Geometry: final body of the model. Coordinates: model frame, mm. Face numbers are marked on the shaded views. A direction names the side the tool comes from. Give positions to 0.01 mm unless a question says otherwise; leave off trailing zeros. Order: outer loops, then holes, each group sorted by start corner. A loop starts at its lowest first (then second) coordinate and runs counter-clockwise, first axis right, second up. Notation, with made-up numbers: (89.5, 13.5) -> (103.5, 13.5) arc R27 ccw to (103.5, 40.5) -> close; hole circle Ø10 at (-36.5, 23). An arc over 180 degrees is marked (long way). One line per question, with ' | ' between items.
from build123d import *

# Parameters (mm, degrees)
ESBO_O1_R                  = 72.5
ESBO_O1_R_2                = 52.5
RESSALTO_EXTRUS_O1_DEPTH   = 50
CORTE_EXTRUS_O1_DEPTH      = 115.072345465
CORTE_EXTRUS_O1_DEPTH_BACK = 115.072345465
ESBO_O2_W                  = 40
ESBO_O2_H                  = 97.356983932
RESSALTO_EXTRUS_O2_START   = -30
ESBO_O3_R                  = 52.5
ESBO_O3_R_2                = 47.8
RESSALTO_EXTRUS_O2_DEPTH   = 30
CORTE_EXTRUS_O2_DEPTH      = 115.072345465
CORTE_EXTRUS_O2_DEPTH_BACK = 115.072345465
ESBO_O5_W                  = 23.143765799
ESBO_O5_H                  = 26
CORTE_EXTRUS_O3_DEPTH      = 115.072345465


with BuildPart() as part:
    # Esboço1 → Ressalto-extrusão1 (new body)
    with BuildSketch(Plane(origin=(0, 0, 0), x_dir=(1, 0, 0), z_dir=(0, 1, 0))):
        with Locations(Location((0, 0, 0), (0, 0, 270))):
            Circle(ESBO_O1_R)
        with Locations(Location((0, 0, 0), (0, 0, 270))):
            Circle(ESBO_O1_R_2, mode=Mode.SUBTRACT)
    extrude(amount=RESSALTO_EXTRUS_O1_DEPTH)

    # Esboço2 → Corte-extrusão1 (cut, two sides: drawn at the far end of the back side and taken through both)
    with BuildSketch(Plane(origin=(0, 50, 0), x_dir=(1, 0, 0), z_dir=(0, 1, 0)).offset(-CORTE_EXTRUS_O1_DEPTH_BACK)):
        with Locations((0, 48.678491966)):
            Rectangle(ESBO_O2_W, ESBO_O2_H)
    extrude(amount=CORTE_EXTRUS_O1_DEPTH + CORTE_EXTRUS_O1_DEPTH_BACK, mode=Mode.SUBTRACT)

    # Esboço3 → Ressalto-extrusão2 (add)
    with BuildSketch(Plane(origin=(0, 50, 0), x_dir=(1, 0, 0), z_dir=(0, 1, 0)).offset(RESSALTO_EXTRUS_O2_START)):
        Circle(ESBO_O3_R)
        with Locations(Location((0, 0, 0), (0, 0, 270))):
            Circle(ESBO_O3_R_2, mode=Mode.SUBTRACT)
    extrude(amount=RESSALTO_EXTRUS_O2_DEPTH)

    # Esboço4 → Corte-extrusão2 (cut, two sides: drawn at the far end of the back side and taken through both)
    with BuildSketch(Plane(origin=(0, 50, 0), x_dir=(1, 0, 0), z_dir=(0, 1, 0)).offset(-CORTE_EXTRUS_O2_DEPTH_BACK)):
        Polygon((-20, 69.686799324), (-20, 29.755386526), (20, 29.755386526), (20, 73.66525197), (-20, 73.66525197), align=None)
    extrude(amount=CORTE_EXTRUS_O2_DEPTH + CORTE_EXTRUS_O2_DEPTH_BACK, mode=Mode.SUBTRACT)

    # Esboço5 → Corte-extrusão3 (cut, through all)
    with BuildSketch(Plane(origin=(0, 0, 0), x_dir=(0, 0, -1), z_dir=(1, 0, 0))):
        with Locations((-61.895664133, 33.904990218)):
            Rectangle(ESBO_O5_W, ESBO_O5_H)
    extrude(amount=-CORTE_EXTRUS_O3_DEPTH, mode=Mode.SUBTRACT)


solid = part.part
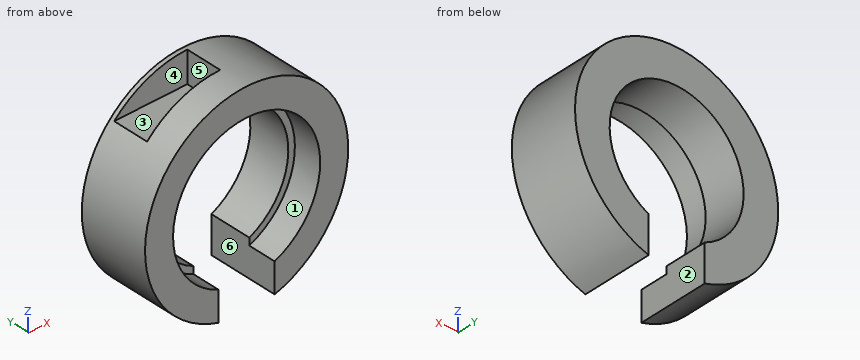
1) Section B-B on y = 44.5. Return loops of the section in (x, z), plus the area to 3 significant figures.
Check result:
outline: (-52.19, 50.32) arc R72.5 ccw to (-20, -69.69) -> (-20, -43.41) arc R47.8 cw (long way) to (20, -43.41) -> (20, -69.69) arc R72.5 ccw to (0, 72.5) -> (0, 50.32) -> close | area: 7,530 mm^2
2) Pull-direction query (X, two-part tool) for the marked faces 4, 5 and 6; classes: +X half, -X half, draft (parallel to the pull), parting line (faces both ways), or undercut.
Check result:
face 4: draft | face 5: -X half | face 6: undercut
3) Contact query for flat-ended pins moving along their axis: pin 1 Ø8 at (y, z) = (18.5, -50.5) entering from +X; pin 2 Ø10 at (x, y) = (-4, 28) entering from +Z; pin 3 Ø6 at (y, z) = (36, -17) entering from +X; pin 4 Ø6 at (x, y) = (5.5, 6) entering from -Z. Output: stop coordinate, or through.
Check result:
pin 1: stops at x = 55.62 | pin 2: stops at z = 72.5 | pin 3: stops at x = 71.14 | pin 4: stops at z = 51.81
4) Section D-D on z = 39.5. Return loops of the section in (x, y), plus the area to 3 significant figures.
Check result:
outline: (-60.79, 0) -> (-34.58, 0) -> (-34.58, 20) -> (-26.92, 20) -> (-26.92, 50) -> (-60.79, 50) -> close; (26.92, 20) -> (34.58, 20) -> (34.58, 0) -> (60.79, 0) -> (60.79, 50) -> (26.92, 50) -> close | area: 3,080 mm^2
5) Section A-A on z = 0. Return loops of the section in (x, y).
Check result:
outline: (-72.5, 0) -> (-52.5, 0) -> (-52.5, 20) -> (-47.8, 20) -> (-47.8, 50) -> (-72.5, 50) -> close; (47.8, 20) -> (52.5, 20) -> (52.5, 0) -> (72.5, 0) -> (72.5, 50) -> (47.8, 50) -> close
6) Material intervals for probe 1 along X at (y, z) = (39.5, 0); probe 2 along X at (y, z) = (12, 0); probe 3 along Z at (x, y) = (0, 16.25), sorted ascending. Write a range as from..to.
Check result:
probe 1: x = -72.5..-47.8, 47.8..72.5 | probe 2: x = -72.5..-52.5, 52.5..72.5 | probe 3: z = 52.5..72.5
7) Section C-C on x = -28. Return loops of the section in (y, z) (3 decimals).
Check result:
outline: (0, -66.875) -> (50, -66.875) -> (50, -38.741) -> (20, -38.741) -> (20, -44.41) -> (0, -44.41) -> close; (0, 44.41) -> (20, 44.41) -> (20, 38.741) -> (50, 38.741) -> (50, 66.875) -> (46.905, 66.875) -> (46.905, 50.324) -> (20.905, 50.324) -> (20.905, 66.875) -> (0, 66.875) -> close
8) Set-up query: the marked faces 1, 2 and 3. Return all of +Z, -Z, +X, -X, +Y, -Y with unobstructed straight access to the full face (end or side cutting, diameter ignored); none if empty.
Check result:
face 1: -Y | face 2: -Z, +Y, -Y | face 3: +Z, -X
